For this review, use the dimensioned drawing (mm, ordinates from the lowest corner) and the shaded views. A direction names the side the tool comes from. Coordinates: 2 decimals unless noted, no trailing zeros. Loops run counter-clockwise (first coordinate to the right, second up) from the corner with the lowest first, then second, coordinate; pieces in that order, holes last. Notation, with made-up numbers: (73, 63) - (127, 63) arc R28 cw to (127, 97) - close; hole circle Ø1 at (-39.5, 60.25). An arc over 180 degrees is marked (long way). Answer in a Markdown table with one row per item. Add a question column.
(1) Mouldability with a two-part tool opening along X and no side actions: class the marked faces 3, 4 and 5 as +X half, -X half, draft (parallel to the pull), parting line (faces both ways), or undercut.
(2) We need section C-C on z = 47.5. Write out the cut boundary in (x, y), plus the area to 3 significant figures.
(3) We need section D-D on x = 13.5. Write out the cut boundary in (y, z), plus the area to 3 significant figures.
(4) Machinability: for the marked faces 1 and 2, which of the approach directions +Z, -Z, +X, -X, +Y, -Y give a long, thin tool a straight path to every point of the face, cutting with its end or side? Answer none if there is none.
(5) We need section B-B on y = 13. Write out the cut boundary in (x, z).
(6) We need section A-A on x = 120. Write out the cut boundary in (y, z), plus the area to 3 significant figures.
(7) For P1, Ø2, axis at y = 31.5, z = 49, coming from the +X side; P2, Ø8, axis at x = 113, y = 16.5, coming from the +Z side; P3, Ø6, axis at y = 33, z = 32.5, coming from the -X side, all flat-tipped, find the tip position at first contact; note any pin that passes through.
(8) For line 1 along Z through (x, y) = (120, 41.5); line 2 along X through (y, z) = (29, 66); line 3 along X through (y, z) = (38, 30), list the stretches that pass through material, from the lowest coordinate up.
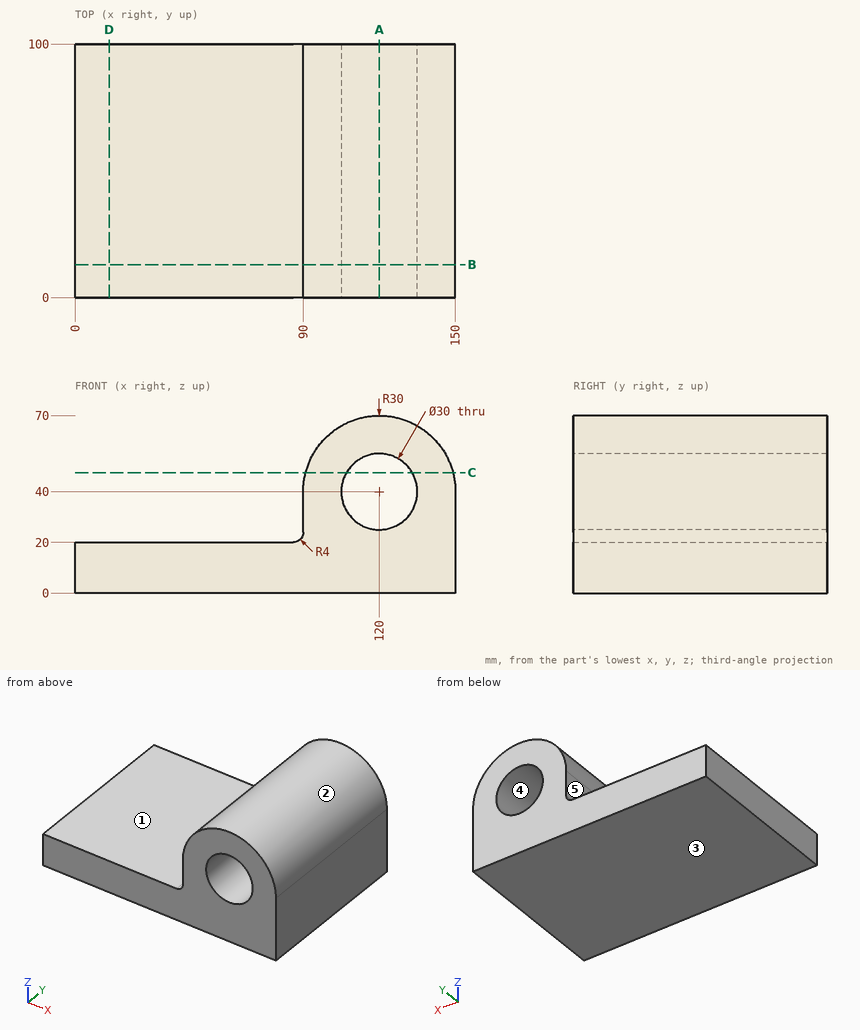
Outcome:
| question | item | result |
|---|---|---|
| 1 | face 3 | draft |
| 1 | face 4 | undercut |
| 1 | face 5 | -X half |
| 2 | outline | (90.95, 0) - (107.01, 0) - (107.01, 100) - (90.95, 100) - close; (132.99, 0) - (149.05, 0) - (149.05, 100) - (132.99, 100) - close |
| 2 | area | 3,210 mm² |
| 3 | outline | (0, 0) - (100, 0) - (100, 20) - (0, 20) - close |
| 3 | area | 2,000 mm² |
| 4 | face 1 | +Z, -X, +Y, -Y |
| 4 | face 2 | +Z, +Y, -Y |
| 5 | outline | (0, 0) - (150, 0) - (150, 40) arc R30 ccw to (90, 40) - (90, 24) arc R4 cw to (86, 20) - (0, 20) - close; hole circle Ø30 at (120, 40) |
| 6 | outline | (0, 0) - (100, 0) - (100, 25) - (0, 25) - close; (0, 55) - (100, 55) - (100, 70) - (0, 70) - close |
| 6 | area | 4,000 mm² |
| 7 | P1 | x = 148.91 |
| 7 | P2 | z = 69.85 |
| 7 | P3 | x = 90 |
| 8 | line 1 | 0 to 25, 55 to 70 |
| 8 | line 2 | 105.03 to 134.97 |
| 8 | line 3 | 90 to 108.82, 131.18 to 150 |
